Build history of the part. All positions in model axes, mm. Face numbers are marked on the shaded views. Give positions to 0.01 mm unless a question says otherwise; leave off trailing zeros. Loops run counter-clockwise (first coordinate to the right, second up) from the corner with the lowest first, then second, coordinate; pieces in that order, holes last. Notation, with made-up numbers: M 87.25,12.25 L 138.25,12.25 A13 ccw 138.25,22.25 Z; hole C 62,27 d7. An arc over 180 degrees is marked long. Answer as a JSON object with one key per item and string values. Group by question number.
1. Mould opens along Z. For the marked faces 1 and 2 say: released by +Z, released by -Z, zero draft, split by the parting line, or undercut.
2. Drill centre lines: line 1 along X through (y, z) = (4.45, 161); line 2 along Z through (x, y) = (97, 4.1); line 3 along Y through (x, z) = (-76, -192.5). Where is each one in solid material? Low to high. Write a range as [from, to].
3. Slice it at B-B (x = 36). List the corners of the cut face in (y, z), then the cut area to 3 significant figures.
4. Slice it at A-A (z = -95). List the corners of the cut face in (x, y), then the cut area to 4 significant figures.
5. Slice it at C-C (y = 4.7). Give the number of separate pieces and of enclosed holes in the cut face, then the cut area to 3 significant figures.
6. Drop flat-ended pins along their axis: pin 1 Ø10 at (x, z) = (-12, 237) entering from +Y; pin 2 Ø5.5 at (x, z) = (-113.93, -74.29) entering from -Y. Give the stop position or say it passes through.
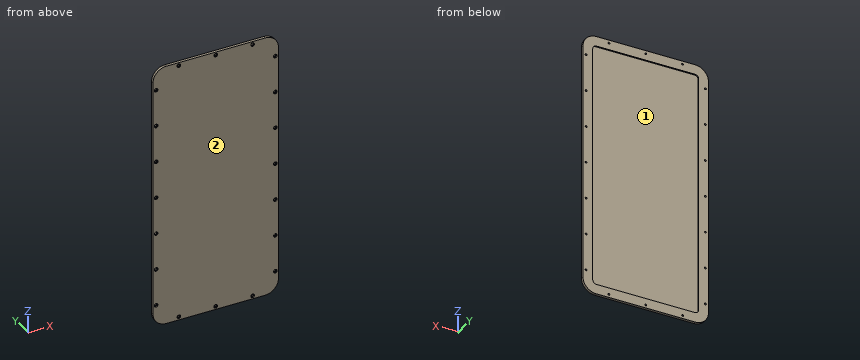
from build123d import *

# Parameters (mm, degrees)
SKETCH1_R           = 2.1
BOSS_EXTRUDE1_DEPTH = 6
CUT_EXTRUDE1_DEPTH  = 3
SKETCH4_R           = 4.125
CUT_EXTRUDE2_DEPTH  = 2.5


with BuildPart() as part:
    # Sketch1 → Boss-Extrude1 (new body)
    with BuildSketch(Plane(origin=(0, 0, 0), x_dir=(-1, 0, 0), z_dir=(0, 1, 0))):
        with BuildLine():
            Line((90.927407972, 302.93116582), (-129.072592028, 302.93116582))
            ThreePointArc((-129.072592028, 302.93116582), (-150.285795463, 294.144369255), (-159.072592028, 272.93116582))
            Line((-159.072592028, 272.93116582), (-159.072592028, -257.06883418))
            ThreePointArc((-159.072592028, -257.06883418), (-150.285795463, -278.282037616), (-129.072592028, -287.06883418))
            Line((-129.072592028, -287.06883418), (90.927407972, -287.06883418))
            ThreePointArc((90.927407972, -287.06883418), (112.140611408, -278.282037616), (120.927407972, -257.06883418))
            Line((120.927407972, -257.06883418), (120.927407972, 272.93116582))
            ThreePointArc((120.927407972, 272.93116582), (112.140611408, 294.144369255), (90.927407972, 302.93116582))
        make_face()
        with Locations((-152.072592028, 254.608155129)):
            Circle(SKETCH1_R, mode=Mode.SUBTRACT)
        with Locations((-101.298255131, 295.93116582)):
            Circle(SKETCH1_R, mode=Mode.SUBTRACT)
        with Locations((-19.072592028, 295.93116582)):
            Circle(SKETCH1_R, mode=Mode.SUBTRACT)
        with Locations((63.153071075, 295.93116582)):
            Circle(SKETCH1_R, mode=Mode.SUBTRACT)
        with Locations((113.927407972, 254.608155129)):
            Circle(SKETCH1_R, mode=Mode.SUBTRACT)
        with Locations((-152.072592028, 7.93116582)):
            Circle(SKETCH1_R, mode=Mode.SUBTRACT)
        with Locations((-152.072592028, -74.294497284)):
            Circle(SKETCH1_R, mode=Mode.SUBTRACT)
        with Locations((-152.072592028, -156.520160387)):
            Circle(SKETCH1_R, mode=Mode.SUBTRACT)
        with Locations((-152.072592028, -238.74582349)):
            Circle(SKETCH1_R, mode=Mode.SUBTRACT)
        with Locations((-101.298255131, -280.06883418)):
            Circle(SKETCH1_R, mode=Mode.SUBTRACT)
        with Locations((-19.072592028, -280.06883418)):
            Circle(SKETCH1_R, mode=Mode.SUBTRACT)
        with Locations((63.153071075, -280.06883418)):
            Circle(SKETCH1_R, mode=Mode.SUBTRACT)
        with Locations((113.927407972, -238.74582349)):
            Circle(SKETCH1_R, mode=Mode.SUBTRACT)
        with Locations((113.927407972, -156.520160387)):
            Circle(SKETCH1_R, mode=Mode.SUBTRACT)
        with Locations((113.927407972, -74.294497284)):
            Circle(SKETCH1_R, mode=Mode.SUBTRACT)
        with Locations((113.927407972, 7.93116582)):
            Circle(SKETCH1_R, mode=Mode.SUBTRACT)
        with Locations((-152.072592028, 90.156828923)):
            Circle(SKETCH1_R, mode=Mode.SUBTRACT)
        with Locations((-152.072592028, 172.382492026)):
            Circle(SKETCH1_R, mode=Mode.SUBTRACT)
        with Locations((113.927407972, 90.156828923)):
            Circle(SKETCH1_R, mode=Mode.SUBTRACT)
        with Locations((113.927407972, 172.382492026)):
            Circle(SKETCH1_R, mode=Mode.SUBTRACT)
    extrude(amount=BOSS_EXTRUDE1_DEPTH)

    # Sketch3 → Cut-Extrude1 (cut)
    with BuildSketch(Plane(origin=(0, 6, 0), x_dir=(1, 0, 0), z_dir=(0, 1, 0))):
        with BuildLine():
            Line((129.072592028, -281.18116582), (-90.927407972, -281.18116582))
            ThreePointArc((-90.927407972, -281.18116582), (-96.761038917, -278.764796764), (-99.177407972, -272.93116582))
            Line((-99.177407972, -272.93116582), (-99.177407972, 257.06883418))
            ThreePointArc((-99.177407972, 257.06883418), (-96.761038917, 262.902465125), (-90.927407972, 265.31883418))
            Line((-90.927407972, 265.31883418), (129.072592028, 265.31883418))
            ThreePointArc((129.072592028, 265.31883418), (134.906222973, 262.902465125), (137.322592028, 257.06883418))
            Line((137.322592028, 257.06883418), (137.322592028, -272.93116582))
            ThreePointArc((137.322592028, -272.93116582), (134.906222973, -278.764796764), (129.072592028, -281.18116582))
        make_face()
    extrude(amount=-CUT_EXTRUDE1_DEPTH, mode=Mode.SUBTRACT)

    # Sketch4 → Cut-Extrude2 (cut)
    with BuildSketch(Plane.XZ):
        with Locations((101.298255131, -280.06883418)):
            Circle(SKETCH4_R)
        with Locations((152.072592028, -238.74582349)):
            Circle(SKETCH4_R)
        with Locations((19.072592028, -280.06883418)):
            Circle(SKETCH4_R)
        with Locations((-63.153071075, -280.06883418)):
            Circle(SKETCH4_R)
        with Locations((-113.927407972, -238.74582349)):
            Circle(SKETCH4_R)
        with Locations((-113.927407972, -156.520160387)):
            Circle(SKETCH4_R)
        with Locations((-113.927407972, -74.294497284)):
            Circle(SKETCH4_R)
        with Locations((-113.927407972, 7.93116582)):
            Circle(SKETCH4_R)
        with Locations((-113.927407972, 90.156828923)):
            Circle(SKETCH4_R)
        with Locations((-113.927407972, 172.382492026)):
            Circle(SKETCH4_R)
        with Locations((-113.927407972, 254.608155129)):
            Circle(SKETCH4_R)
        with Locations((-63.153071075, 295.93116582)):
            Circle(SKETCH4_R)
        with Locations((19.072592028, 295.93116582)):
            Circle(SKETCH4_R)
        with Locations((101.298255131, 295.93116582)):
            Circle(SKETCH4_R)
        with Locations((152.072592028, 254.608155129)):
            Circle(SKETCH4_R)
        with Locations((152.072592028, 172.382492026)):
            Circle(SKETCH4_R)
        with Locations((152.072592028, 90.156828923)):
            Circle(SKETCH4_R)
        with Locations((152.072592028, 7.93116582)):
            Circle(SKETCH4_R)
        with Locations((152.072592028, -74.294497284)):
            Circle(SKETCH4_R)
        with Locations((152.072592028, -156.520160387)):
            Circle(SKETCH4_R)
    extrude(amount=-CUT_EXTRUDE2_DEPTH, mode=Mode.SUBTRACT)


solid = part.part
Established:
{
 "1": {"face 1": "undercut", "face 2": "zero draft"},
 "2": {"line 1": "x = [-120.93, -99.18], [137.32, 159.07]", "line 2": "z = [-287.07, -265.32], [281.18, 302.93]", "line 3": "y = [0, 3]"},
 "3": {"outline": "M 0,-287.07 L 6,-287.07 L 6,-265.32 L 3,-265.32 L 3,281.18 L 6,281.18 L 6,302.93 L 0,302.93 Z", "area": "1,900 mm^2"},
 "4": {"outline": "M -120.93,0 L 159.07,0 L 159.07,6 L 137.32,6 L 137.32,3 L -99.18,3 L -99.18,6 L -120.93,6 Z", "area": "970.5 mm^2"},
 "5": {"separate pieces": "1", "enclosed holes": "21", "area": "35,000 mm^2"},
 "6": {"pin 1": "stops at y = 3", "pin 2": "stops at y = 2.5"}
}
